For this review, take the finished solid that the model builds, in its own axes (mm). Face numbers are marked on the shaded views. A direction names the side the tool comes from. Round coordinates to 2 decimals unless told otherwise and drop trailing zeros. Write each loop counter-clockwise with the first axis right and the second up, starting at its lowest first coordinate (ties: lowest second). Pieces come first, ordered by that corner, then holes. Notation, with made-up numbers: (64.5, 78.25) - (81.5, 78.25) arc R19 ccw to (81.5, 103.25) - close; hole circle Ø11 at (44.5, 33). An arc over 180 degrees is marked (long way). One line per item, written item: value. Start each with the question number.
Q1. Mouldability with a two-part tool opening along X and no side actions: class the marked faces 1, 2 and 3 as +X half, -X half, draft (parallel to the pull), parting line (faces both ways), or undercut.
Q2. Clearance check with flat-ended pins moving along their axes: pin 1 Ø1 at (x, z) = (18.5, 23) entering from +Y; pin 2 Ø8 at (x, z) = (15.5, 17) entering from -Y. State where each tip first meets the part, or that it passes through.
Q3. Add section B-B on z = 6. Write out the cut boundary in (x, y), and give its area (3 significant figures).
Q4. Tool access review of the marked faces 4, 5 and 6: name each direction out of +Z, -Z, +X, -X, +Y, -Y from which nothing blocks a thin tool from reaching the whole face with its end or side.
Q5. Add section C-C on y = 21. Write out the cut boundary in (x, z).
Q6. Add section A-A on y = 56. Write out the cut boundary in (x, z).
Q7. For probe 1 along X at (y, z) = (43, 9); probe 2 along X at (y, z) = (16, 54); probe 3 along Y at (x, z) = (8, 13.5), list the stretches that pass through material, from the lowest coordinate up.
Q8. Add section D-D on x = 9. Write out the cut boundary in (y, z).
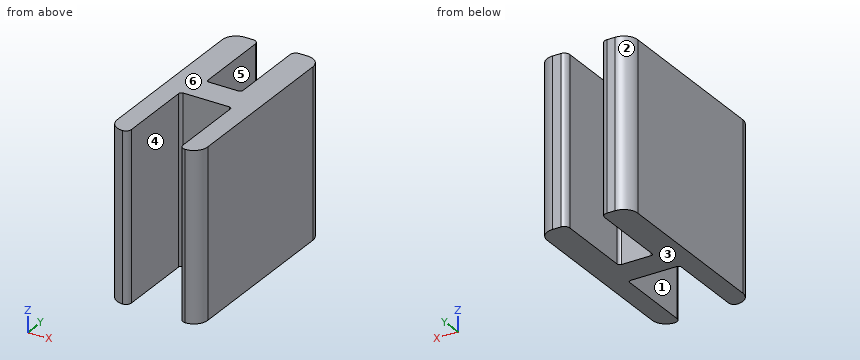
```python
from build123d import *

# Parameters (mm, degrees)
F1_DEPTH = 60


with BuildPart() as f1:
    # F0 (on Top) → F1 (new body)
    with BuildSketch(Plane.XY):
        with BuildLine():
            Line((0, 65), (0, 5))
            ThreePointArc((0, 5), (1.464466, 1.464466), (5, 0))
            ThreePointArc((5, 0), (6.414214, 0.585786), (7, 2))
            Line((7, 2), (7, 29))
            ThreePointArc((7, 29), (7.292893, 29.707107), (8, 30))
            Line((8, 30), (24.5, 30))
            ThreePointArc((24.5, 30), (25.207107, 29.707107), (25.5, 29))
            Line((25.5, 29), (25.5, 2))
            ThreePointArc((25.5, 2), (26.085786, 0.585786), (27.5, 0))
            ThreePointArc((27.5, 0), (31.035534, 1.464466), (32.5, 5))
            Line((32.5, 5), (32.5, 65))
            ThreePointArc((32.5, 65), (31.035534, 68.535534), (27.5, 70))
            Line((27.5, 70), (24.5, 70))
            ThreePointArc((24.5, 70), (23.085786, 69.414214), (22.5, 68))
            Line((22.5, 68), (22.5, 41))
            ThreePointArc((22.5, 41), (22.207107, 40.292893), (21.5, 40))
            Line((21.5, 40), (11, 40))
            ThreePointArc((11, 40), (10.292893, 40.292893), (10, 41))
            Line((10, 41), (10, 68))
            ThreePointArc((10, 68), (9.414214, 69.414214), (8, 70))
            Line((8, 70), (5, 70))
            ThreePointArc((5, 70), (1.464466, 68.535534), (0, 65))
        make_face()
    extrude(amount=F1_DEPTH)


solid = f1.part
```
Result set:
1. face 1: undercut
1. face 2: -X half
1. face 3: draft
2. pin 1: stops at y = 40
2. pin 2: stops at y = 30
3. outline: (0, 5) arc R5 ccw to (5, 0) arc R2 ccw to (7, 2) - (7, 29) arc R1 cw to (8, 30) - (24.5, 30) arc R1 cw to (25.5, 29) - (25.5, 2) arc R2 ccw to (27.5, 0) arc R5 ccw to (32.5, 5) - (32.5, 65) arc R5 ccw to (27.5, 70) - (24.5, 70) arc R2 ccw to (22.5, 68) - (22.5, 41) arc R1 cw to (21.5, 40) - (11, 40) arc R1 cw to (10, 41) - (10, 68) arc R2 ccw to (8, 70) - (5, 70) arc R5 ccw to (0, 65) - close
3. area: 1,320 mm^2
4. face 4: +Z, -Z, -Y
4. face 5: +Z, -Z, +Y
4. face 6: +Z, +X, -X, +Y, -Y
5. outline: (0, 0) - (7, 0) - (7, 60) - (0, 60) - close; (25.5, 0) - (32.5, 0) - (32.5, 60) - (25.5, 60) - close
6. outline: (0, 0) - (10, 0) - (10, 60) - (0, 60) - close; (22.5, 0) - (32.5, 0) - (32.5, 60) - (22.5, 60) - close
7. probe 1: x = 0 to 10, 22.5 to 32.5
7. probe 2: x = 0 to 7, 25.5 to 32.5
7. probe 3: y = 30 to 70
8. outline: (30, 0) - (69.73, 0) - (69.73, 60) - (30, 60) - close
